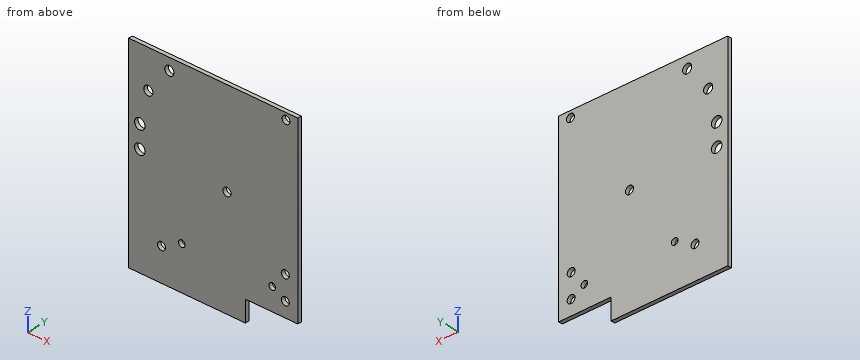
from build123d import *

# Parameters (mm, degrees)
F1_DEPTH = 3
F2_D     = 7
F3_D     = 6.1
F4_D     = 6
F6_D     = 5
F7_D     = 8
F8_D     = 6


with BuildPart() as f1:
    # F0 (on Front) → F1 (new body)
    with BuildSketch(Plane.XZ):
        Polygon((129, 0), (0, 0), (0, -154), (89, -154), (89, -138), (129, -138), align=None)
    extrude(amount=F1_DEPTH)

    # F2 (through all)
    with Locations(Plane(origin=(0, 0, 0), x_dir=(1, 0, 0), z_dir=(0, 1, 0))):
        with Locations((15, 29), (31, 9)):
            Hole(F2_D / 2)

    # F3 (through all)
    with Locations(Plane(origin=(0, 0, 0), x_dir=(1, 0, 0), z_dir=(0, 1, 0))):
        with Locations((75, 72)):
            Hole(F3_D / 2)

    # F4 (through all)
    with Locations(Plane(origin=(0, 0, 0), x_dir=(1, 0, 0), z_dir=(0, 1, 0))):
        with Locations((120, 5), (25, 129)):
            Hole(F4_D / 2)

    # F6 (through all)
    with Locations(Plane.XZ.offset(3)):
        with Locations((40.5317286446, -120.9223137817), (109.4682713554, -120.9223137817)):
            Hole(F6_D / 2)

    # F7 (through all)
    with Locations(Plane.XZ.offset(3)):
        with Locations((8.5, -71), (8.5, -54)):
            Hole(F7_D / 2)

    # F8 (through all)
    with Locations(Plane.XZ.offset(3)):
        with Locations((119.5, -108.667), (119.5, -126.667)):
            Hole(F8_D / 2)


solid = f1.part
Geometry check sheet. Reference: the model listing, model coordinates, mm. Round coordinates to 2 decimals unless told otherwise and drop trailing zeros. Loops run counter-clockwise (first coordinate to the right, second up) from the corner with the lowest first, then second, coordinate; pieces in that order, holes last.
Item 1: Gauge pin test, flat end, axial feed: pin 1 (5 mm diameter, centred on x = 8.5, z = -54, fed in from -Y). Record the tip position at first contact, or that the pin passes through.
Item 2: Cross-section at A-A on x = 75. Record the boundary of the cut face in (y, z).
Item 3: Cross-section at B-B on z = -29. Record the boundary of the cut face in (x, y).
Item 4: Thickness scan on line 1 (Z direction, x = 8.5, y = -0.55); line 2 (Z direction, x = 120, y = -1.05); line 3 (Z direction, x = 40.5, y = -0.85). Record the ranges inside material, lowest first.
Item 5: Cross-section at D-D on y = -1.5. Count the separate pieces of the cut face and the enclosed holes in it, then the cut area to 3 significant figures.
Item 6: Cross-section at C-C on x = 120. Record the boundary of the cut face in (y, z), then the cut area to 3 significant figures.
Answer sheet:
1. pin 1: passes through
2. outline: (-3, -154) - (0, -154) - (0, -75.05) - (-3, -75.05) - close; (-3, -68.95) - (0, -68.95) - (0, 0) - (-3, 0) - close
3. outline: (0, -3) - (11.5, -3) - (11.5, 0) - (0, 0) - close; (18.5, -3) - (129, -3) - (129, 0) - (18.5, 0) - close
4. line 1: z = -154 to -75, -67 to -58, -50 to 0
4. line 2: z = -138 to -129.63, -123.71 to -111.63, -105.71 to -8, -2 to 0
4. line 3: z = -154 to -123.42, -118.42 to 0
5. separate pieces: 1
5. enclosed holes: 11
5. area: 18,900 mm2
6. outline: (-3, -138) - (0, -138) - (0, -129.63) - (-3, -129.63) - close; (-3, -123.71) - (0, -123.71) - (0, -111.63) - (-3, -111.63) - close; (-3, -105.71) - (0, -105.71) - (0, -8) - (-3, -8) - close; (-3, -2) - (0, -2) - (0, 0) - (-3, 0) - close
6. area: 361 mm2
